Geometry: see drawing. Coordinates: mm, zero at the bounding-box minimum. Round coordinates to 2 decimals unless told otherwise and drop trailing zeros. Loops run counter-clockwise (first coordinate to the right, second up) from the corner with the lowest first, then second, coordinate; pieces in that order, holes last. Notation, with made-up numbers: (63, 72) - (67, 72) arc R4 cw to (67, 76) - close; hole circle Ø5 at (80, -3). An arc over 180 degrees is marked (long way). Write item = value, one per line. Start each with the question number.
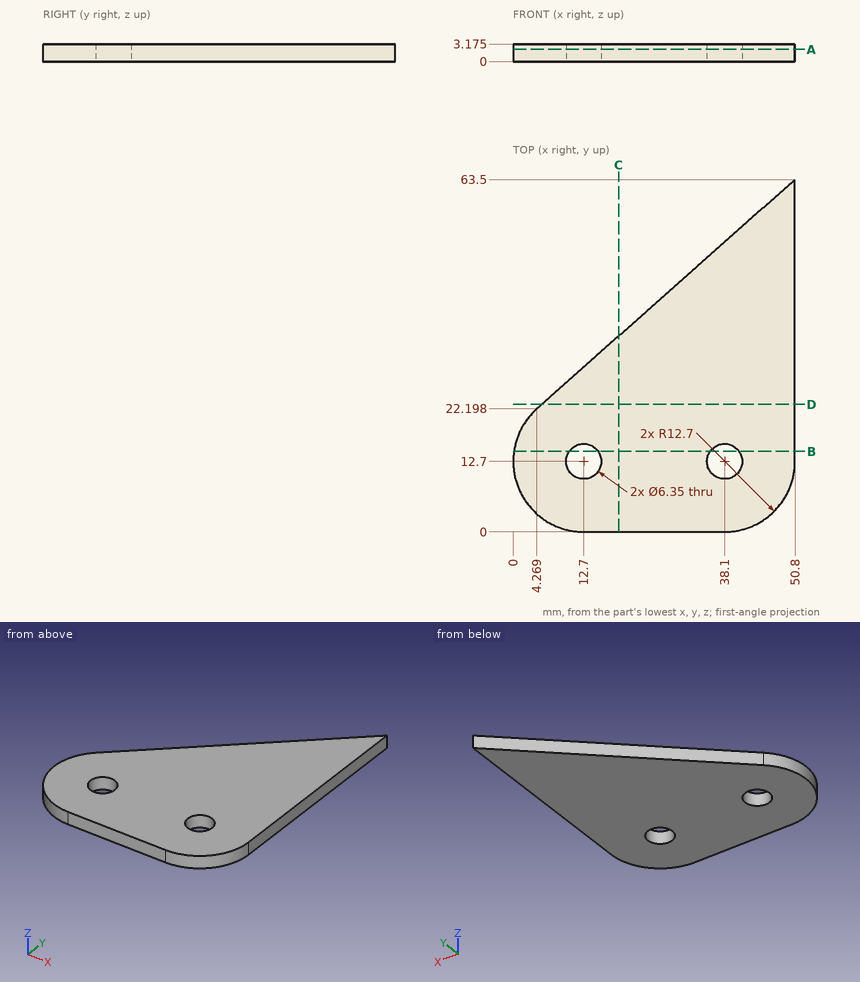
(1) Cut plane A-A (z = 2.2). State how many separate pieces and enclosed holes the cut face has, and give its area (3 significant figures).
(2) Cut plane C-C (x = 19). Output: boundary loops of the cut face in (y, z) (1 decimal).
(3) Cut plane B-B (y = 14.5). Output: boundary loops of the cut face in (x, z) (1 decimal).
(4) Material intervals for line 1 along Y through (x, z) = (12.7, 0.9) (1 decimal); line 2 along Y through (x, z) = (22.5, 2.25); line 3 along X through (y, z) = (55, 0.75) (1 decimal), sorted ascending. Write a range as from..to.
(5) Cut plane D-D (y = 23). Output: boundary loops of the cut face in (x, z) (1 decimal), and give its area (3 significant figures).
Solution:
q1.separate_pieces = 1
q1.enclosed_holes = 2
q1.area = 1,940 mm^2
q2.outline = (0, 0) - (35.3, 0) - (35.3, 3.2) - (0, 3.2) - close
q3.outline = (0.1, 0) - (10.1, 0) - (10.1, 3.2) - (0.1, 3.2) - close; (15.3, 0) - (35.5, 0) - (35.5, 3.2) - (15.3, 3.2) - close; (40.7, 0) - (50.8, 0) - (50.8, 3.2) - (40.7, 3.2) - close
q4.line_1 = 0..9.5, 15.9..29.7
q4.line_2 = 0..38.38
q4.line_3 = 41.2..50.8
q5.outline = (5.2, 0) - (50.8, 0) - (50.8, 3.2) - (5.2, 3.2) - close
q5.area = 145 mm^2
